Check sheet for the modelled part. Datum: model origin and axes. Units: mm. A direction names the side the tool comes from. Coordinates: 2 decimals unless noted, no trailing zeros. Loops run counter-clockwise (first coordinate to the right, second up) from the corner with the lowest first, then second, coordinate; pieces in that order, holes last. Notation, with made-up numbers: (56, 70.5) - (98, 70.5) arc R33 cw to (98, 98.5) - close; hole circle Ø6 at (35, 47.25). An arc over 180 degrees is marked (long way). Answer as a JSON object with one key per item and string values. Group by question number.
Autodesk Inventor part; units mm, degrees
ref_plane "YZ Plane" through (0, 0, 0) normal (1, 0, 0) x (0, 1, 0)
ref_plane "XZ Plane" through (0, 0, 0) normal (0, 1, 0) x (-1, 0, 0)
ref_plane "XY Plane" through (0, 0, 0) normal (0, 0, 1) x (1, 0, 0)
sketch "Эскиз1" plane through (0, 0, 0) normal (0, 0, 1) x (1, 0, 0)
  line L0 (0, 0) -> (6.5, 0)
  line L1 (6.5, 0) -> (6.5, 2.5)
  line L2 (6.5, 2.5) -> (4.65, 2.5)
  line L3 (4.65, 2.5) -> (4.65, 49.5)
  line L4 (4.65, 49.5) -> (4.55, 49.5)
  line L5 (4.55, 49.5) -> (4.55, 66.5)
  line L6 (4.55, 66.5) -> (0, 66.5)
  line L7 (0, 66.5) -> (0, 0)
  dimension "d1" = 64
  dimension "d2" = 9.3
  dimension "d3" = 0.1
  dimension "d4" = 13
  dimension "d5" = 2.5
  dimension "d6" = 17
revolve "Вращение1" add sketch "Эскиз1" angle 360 about axis through (0, 66.5, 0) along (0, -1, 0)
fillet "Сопряжение1" radius 0.5 2 edges at (-6.5, 2.5, 0) (-6.5, 0, 0)
chamfer "Фаска1" distance 0.5 angle 45 1 edges at (-4.55, 66.5, 0)
properties part number "paris_kingpin"
1. Sectioned sample at C-C on y = 14.5. Record the cut outline in (x, z).
2. Material ranges on line 1 (Y direction, x = 1, z = 4.75); line 2 (Z direction, x = 0, y = 48); line 3 (X direction, y = 48, z = -1), recorded low to high.
3. Gauge pin test, flat ends, axial feed: pin 1 (6 mm diameter, centred on x = -0.5, y = 24, fed in from +Z); pin 2 (6 mm diameter, centred on x = 2.5, y = 11, fed in from -Z); pin 3 (1.5 mm diameter, centred on y = 15, z = -4, fed in from +X). Record the tip position at first contact, or that the pin passes through.
4. Access from +Z, -Z, +X, -X, +Y, -Y to the whole of each face (thin tool, end or side, straight path). Record for faces 1 (the face through (3, 2.5, -4)), 2 (the face through (-5.158, 1.26, 3.955)).
5. Sectioned sample at A-A on z = 0. Record the cut outline in (x, y).
6. Sectioned sample at B-B on x = 0. Record the cut outline in (y, z), plus the area to 3 significant figures.
Answers follow:
{
 "1": {"outline": "circle Ø9.3 at (0, 0)"},
 "2": {"line 1": "y = 0 to 2.5", "line 2": "z = -4.65 to 4.65", "line 3": "x = -4.54 to 4.54"},
 "3": {"pin 1": "stops at z = 4.65", "pin 2": "stops at z = -4.65", "pin 3": "stops at x = 3.33"},
 "4": {"face 1": "+Y", "face 2": "+Y, -Y"},
 "5": {"outline": "(-6.5, 0.5) arc R0.5 ccw to (-6, 0) - (6, 0) arc R0.5 ccw to (6.5, 0.5) - (6.5, 2) arc R0.5 ccw to (6, 2.5) - (4.65, 2.5) - (4.65, 49.5) - (4.55, 49.5) - (4.55, 66) - (4.05, 66.5) - (-4.05, 66.5) - (-4.55, 66) - (-4.55, 49.5) - (-4.65, 49.5) - (-4.65, 2.5) - (-6, 2.5) arc R0.5 ccw to (-6.5, 2) - close"},
 "6": {"outline": "(0, -6) arc R0.5 ccw to (0.5, -6.5) - (2, -6.5) arc R0.5 ccw to (2.5, -6) - (2.5, -4.65) - (49.5, -4.65) - (49.5, -4.55) - (66, -4.55) - (66.5, -4.05) - (66.5, 4.05) - (66, 4.55) - (49.5, 4.55) - (49.5, 4.65) - (2.5, 4.65) - (2.5, 6) arc R0.5 ccw to (2, 6.5) - (0.5, 6.5) arc R0.5 ccw to (0, 6) - close", "area": "624 mm^2"}
}
